Verification items for the finished model (mm, model axes). A direction names the side the tool comes from. Round coordinates to 2 decimals unless told otherwise and drop trailing zeros. Write each loop counter-clockwise with the first axis right and the second up, starting at its lowest first coordinate (ties: lowest second). Pieces come first, ordered by that corner, then holes.
from build123d import *

# Parameters (mm, degrees)
SKETCH1_W           = 52.5
SKETCH1_H           = 105
BOSS_EXTRUDE1_DEPTH = 65
SKETCH2_W           = 97
SKETCH2_H           = 61
CUT_EXTRUDE1_DEPTH  = 48.5
SKETCH4_W           = 8
SKETCH4_H           = 57
CUT_EXTRUDE2_DEPTH  = 2
SKETCH5_W           = 8
SKETCH5_H           = 57
CUT_EXTRUDE3_DEPTH  = 2
SKETCH7_W           = 101
SKETCH7_H           = 8
CUT_EXTRUDE5_DEPTH  = 2
CUT_EXTRUDE6_REACH  = 52.5
SKETCH9_R           = 1.55
SKETCH10_R          = 1.55
CUT_EXTRUDE7_DEPTH  = 104
SKETCH12_W          = 8
SKETCH12_H          = 12
SKETCH12_H_2        = 10
SKETCH12_H_3        = 15
BOSS_EXTRUDE2_DEPTH = 2
SKETCH13_W          = 8
SKETCH13_H          = 12
SKETCH13_H_2        = 15
SKETCH13_H_3        = 10
BOSS_EXTRUDE3_DEPTH = 2


with BuildPart() as part:
    # Sketch1 → Boss-Extrude1 (new body)
    with BuildSketch(Plane(origin=(0, 0, 0), x_dir=(1, 0, 0), z_dir=(0, 1, 0))):
        Rectangle(SKETCH1_W, SKETCH1_H)
    extrude(amount=BOSS_EXTRUDE1_DEPTH)

    # Sketch2 → Cut-Extrude1 (cut)
    with BuildSketch(Plane(origin=(26.25, 0, 0), x_dir=(0, 0, -1), z_dir=(1, 0, 0))):
        with Locations((0, 34.5)):
            Rectangle(SKETCH2_W, SKETCH2_H)
    extrude(amount=-CUT_EXTRUDE1_DEPTH, mode=Mode.SUBTRACT)

    # Sketch4 → Cut-Extrude2 (cut)
    with BuildSketch(Plane(origin=(0, 0, -52.5), x_dir=(-1, 0, 0), z_dir=(0, 0, -1))):
        with Locations((-22.25, 28.5)):
            Rectangle(SKETCH4_W, SKETCH4_H)
        Polygon((26.25, 65), (-26.25, 65), (-26.25, 57), (-18.25, 57), (26.25, 57), align=None)
    extrude(amount=-CUT_EXTRUDE2_DEPTH, mode=Mode.SUBTRACT)

    # Sketch5 → Cut-Extrude3 (cut)
    with BuildSketch(Plane.XY.offset(52.5)):
        Polygon((26.25, 57), (26.25, 65), (-26.25, 65), (-26.25, 57), (18.25, 57), align=None)
        with Locations((22.25, 28.5)):
            Rectangle(SKETCH5_W, SKETCH5_H)
    extrude(amount=-CUT_EXTRUDE3_DEPTH, mode=Mode.SUBTRACT)

    # Sketch7 → Cut-Extrude5 (cut)
    with BuildSketch(Plane.ZY.offset(26.25)):
        with Locations((0, 61)):
            Rectangle(SKETCH7_W, SKETCH7_H)
    extrude(amount=-CUT_EXTRUDE5_DEPTH, mode=Mode.SUBTRACT)

    # Sketch9 → Cut-Extrude6 (cut, up to next)
    with BuildSketch(Plane.ZY.offset(24.25), mode=Mode.PRIVATE) as cut_extrude6_sk1:
        with Locations((0, 61)):
            Circle(SKETCH9_R)
    cut_extrude6_tool1 = extrude(cut_extrude6_sk1.sketch, amount=-CUT_EXTRUDE6_REACH, mode=Mode.PRIVATE) & part.part
    add(cut_extrude6_tool1.solids().sort_by_distance((-24.25, 61, 0))[0], mode=Mode.SUBTRACT)

    # Sketch10 → Cut-Extrude7 (cut, through all)
    with BuildSketch(Plane.XY.offset(50.5)):
        with Locations((22.25, 15)):
            Circle(SKETCH10_R)
        with Locations((22.25, 40)):
            Circle(SKETCH10_R)
    extrude(amount=-CUT_EXTRUDE7_DEPTH, mode=Mode.SUBTRACT)

    # Sketch12 → Boss-Extrude2 (add)
    with BuildSketch(Plane.XY.offset(50.5)):
        with Locations((22.25, 51)):
            Rectangle(SKETCH12_W, SKETCH12_H)
        with Locations((22.25, 5)):
            Rectangle(SKETCH12_W, SKETCH12_H_2)
        with Locations((22.25, 27.5)):
            Rectangle(SKETCH12_W, SKETCH12_H_3)
    extrude(amount=BOSS_EXTRUDE2_DEPTH)

    # Sketch13 → Boss-Extrude3 (add)
    with BuildSketch(Plane(origin=(0, 0, -50.5), x_dir=(-1, 0, 0), z_dir=(0, 0, -1))):
        with Locations((-22.25, 51)):
            Rectangle(SKETCH13_W, SKETCH13_H)
        with Locations((-22.25, 27.5)):
            Rectangle(SKETCH13_W, SKETCH13_H_2)
        with Locations((-22.25, 5)):
            Rectangle(SKETCH13_W, SKETCH13_H_3)
    extrude(amount=BOSS_EXTRUDE3_DEPTH)


solid = part.part
Q1. Sectioned sample at B-B (y = 40). Enter the section's corners in (x, z).
Recorded:
outline: (-26.25, -52.5) - (18.25, -52.5) - (18.25, -50.5) - (20.7, -50.5) - (20.7, -48.5) - (-22.25, -48.5) - (-22.25, 48.5) - (20.7, 48.5) - (20.7, 50.5) - (18.25, 50.5) - (18.25, 52.5) - (-26.25, 52.5) - close; (23.8, -50.5) - (26.25, -50.5) - (26.25, -48.5) - (23.8, -48.5) - close; (23.8, 48.5) - (26.25, 48.5) - (26.25, 50.5) - (23.8, 50.5) - close
Q2. Release check for a two-part mould opening along Z. For faces 1 (the flat face through (-22.25, 35, 1)), 2 (the flat face through (26.25, 3, -4)), 3 (the flat face through (24, 40, 50.5)) record: released by +Z, released by -Z, zero draft, split by the parting line, or undercut.
Recorded:
face 1: undercut
face 2: zero draft
face 3: released by +Z
Q3. Material ranges on line 1 along Y through (x, z) = (22.25, 49.1); line 2 along Z through (x, y) = (22, 55); line 3 along Y through (x, z) = (5, 7), recorded low to high.
Recorded:
line 1: y = 0 to 13.45, 16.55 to 38.45, 41.55 to 65
line 2: z = -52.5 to -48.5, 48.5 to 52.5
line 3: y = 0 to 4
Q4. Tool access check on faces 4 (the flat face through (-24.25, 59, -1)), 5 (the flat face through (20.5, 40.1, -50.5)), 6 (the flat face through (1, 61, -50.5)), 7 (the flat face through (24, 15, 50.5)), 8 (the flat face through (2, 4, 1)). Record the directions out of +Z, -Z, +X, -X, +Y, -Y that give a thin tool (end or side, any length) a straight path to the whole face; none if there is none.
Recorded:
face 4: +Z, -Z, -X, +Y
face 5: -Z, +X
face 6: -Z, +X, -X, +Y
face 7: +Z, +X
face 8: +X, +Y
Q5. Sectioned sample at D-D (x = 22.25). Give the number of separate pieces and of enclosed holes in the cut face, plus the area to 3 significant figures.
Recorded:
separate pieces: 5
enclosed holes: 0
area: 771 mm2
Q6. Sectioned sample at C-C (x = -4). Enter the section's corners in (y, z), plus the area to 3 significant figures.
Recorded:
outline: (0, -52.5) - (57, -52.5) - (57, -50.5) - (65, -50.5) - (65, -48.5) - (4, -48.5) - (4, 48.5) - (65, 48.5) - (65, 50.5) - (57, 50.5) - (57, 52.5) - (0, 52.5) - close
area: 876 mm2
Q7. Depth check by flat-ended pin: P1, Ø2, axis at y = 28.5, z = -4, coming from the +X side; P2, Ø1.6, axis at x = 23, z = -52, coming from the +Y side; P3, Ø12, axis at x = -7, z = -39.5, coming from the +Y side. Enter the tip coordinate at first touch or a pass-through.
Recorded:
P1: stops at x = -22.25
P2: stops at y = 57
P3: stops at y = 4
Q8. Sectioned sample at A-A (y = 61). Enter the section's corners in (x, z).
Recorded:
outline: (-24.25, -50.5) - (26.25, -50.5) - (26.25, -48.5) - (-22.25, -48.5) - (-22.25, -1.55) - (-24.25, -1.55) - close; (-24.25, 1.55) - (-22.25, 1.55) - (-22.25, 48.5) - (26.25, 48.5) - (26.25, 50.5) - (-24.25, 50.5) - close
